Autodesk Inventor part; units mm, degrees
ref_plane "Work Plane1" through (0, 38.1, 0) normal (0, 1, 0) x (-1, 0, 0)
ref_plane "YZ Plane" through (0, 0, 0) normal (1, 0, 0) x (0, 1, 0)
ref_plane "XY Plane" through (0, 0, 0) normal (0, 0, 1) x (1, 0, 0)
sketch "Sketch6" plane through (0, 0, 0) normal (0, 1, 0) x (-1, 0, 0)
  line L0 (0, 0) -> (5.588, 0)
  line L1 (5.588, 0) -> (5.588, -6.35)
  line L2 (5.588, -6.35) -> (0, -6.35)
  line L3 (0, -6.35) -> (0, 0)
  arc A0 (0, -6.35) -> (5.588, -6.35) centre (2.794, -6.35) ccw
  dimension "d25" = 5.588
  dimension "d26" = 6.35
ref_plane "Work Plane1" through (0, 38.1, 0) normal (0, 1, 0) x (-1, 0, 0)
sketch "Sketch8" plane through (0, 38.1, 0) normal (0, 1, 0) x (-1, 0, 0)
  line L0 (4.3815, 0) -> (1.2065, 0)
  line L1 (1.2065, 0) -> (1.2065, -3.81)
  line L2 (1.2065, -3.81) -> (4.3815, -3.81)
  line L3 (4.3815, -3.81) -> (4.3815, 0)
  arc A0 (1.2065, -3.81) -> (4.3815, -3.81) centre (2.794, -3.81) ccw
  point P0 (0, 0)
  dimension "d27" = 3.175
  dimension "d28" = 3.81
  dimension "d49" = 1.2065
loft "Loft1" add profiles "Sketch6", "Sketch8"
sketch "Sketch9" plane through (-5.588, 0, 0) normal (0, 0, 1) x (1, 0, 0)
  line L0 (0, 0) -> (5.588, 0)
  line L1 (5.588, 0) -> (4.3815, 38.1)
  line L2 (1.2065, 38.1) -> (4.3815, 38.1)
  line L3 (0, 0) -> (1.2065, 38.1)
  line L4 (4.3815, 38.1) -> (5.588, 0)
  line L5 (4.5826, 31.75) -> (1.0054, 31.75)
  line L6 (0, 0) -> (1.2065, 38.1)
  dimension "d34" = 6.35
extrude "Extrusion5" add sketch "Sketch9" along normal blind 38.608 contours L3 L2 L1 L5
fillet "Fillet2" radius 1.5875 1 edges at (-2.794, 31.75, 0)
sketch "Sketch12" plane through (-2.794, 0, -6.35) normal (0, -1, 0) x (1, 0, 0)
  circle A0 centre (0, 1.9685) radius 1.27
  arc A1 (-2.794, 0) -> (2.794, 0) centre (0, 0) ccw
  line L0 (0, -2.794) -> (0, 1.9685)
  point P0 (2.794, 6.35)
  dimension "d44" = 2.54
  dimension "d46" = 4.7625
extrude "Extrusion8" cut sketch "Sketch12" against normal blind 10.16
properties part number "RudderStabilizingFinBottom"
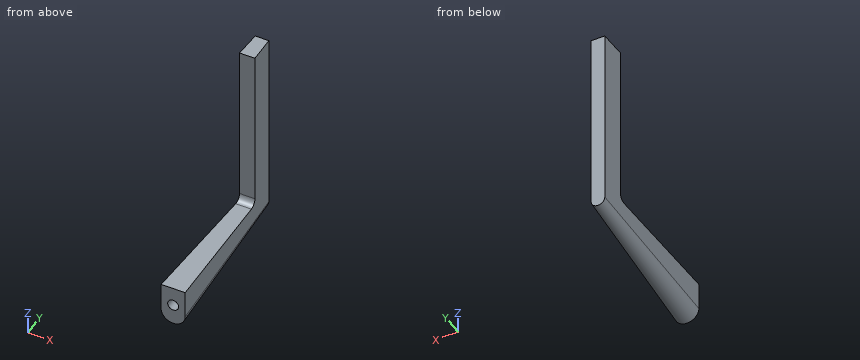
The model under review builds one solid part; all positions refer to its coordinate system, in mm. Give positions to 0.01 mm unless a question says otherwise; leave off trailing zeros. Loops run counter-clockwise (first coordinate to the right, second up) from the corner with the lowest first, then second, coordinate; pieces in that order, holes last. Notation, with made-up numbers: (80, -6.5) -> (116, -6.5) arc R35 ccw to (116, 30.5) -> close; hole circle Ø7 at (3.5, -9.5). An arc over 180 degrees is marked (long way). Put each result on its own line as item: value. Start each with the question number.
1. We need section A-A on z = -1.5. State the section outline as (x, y) points.
2. Clearance check with flat-ended pins moving along their axes: P1, Ø2, axis at x = -4.5, z = 23, coming from the -Y side; P2, Ø2, axis at x = -2.79, z = -4.38, coming from the -Y side. State where each tip first meets the part, or that it passes through.
3. We need section B-B on z = 36.5. State the section outline as (x, y) points, then the cut area to 3 significant figures.
4. Wall thickness on probe 1 along Y at (x, z) = (-2.2, 9); probe 2 along Z at (x, y) = (-2.7, 10); probe 3 along Z at (x, y) = (-3.9, 8): over which ranges is each line inside the solid? List them lowest first.
Determined:
1. outline: (-5.59, 0) -> (0, 0) -> (-1.21, 38.1) -> (-4.38, 38.1) -> close
2. P1: y = 31.75
2. P2: y = 10.16
3. outline: (-4.58, 31.75) -> (-1.01, 31.75) -> (-1.21, 38.1) -> (-4.38, 38.1) -> close
3. area: 21.4 mm^2
4. probe 1: 31.75 to 38.1
4. probe 2: -8.16 to -5.65, -3.11 to 0
4. probe 3: -8.1 to -5.01, -3.76 to 0
